Input: dimensioned drawing with shaded views. Units: mm. Origin: part minimum x, y, z. A direction names the side the tool comes from. Give positions to 0.01 mm unless a question says otherwise; leave off trailing zeros. Write each loop counter-clockwise with the first axis right and the second up, starting at its lowest first coordinate (ties: lowest second). Pieces come first, ordered by that corner, then holes. Notation, with made-up numbers: (4, 78.5) - (48, 78.5) arc R14 cw to (48, 102.5) - close; hole circle Ø4 at (39, 41.5). An arc over 180 degrees is marked (long way). Answer as CSV lines item,"result".
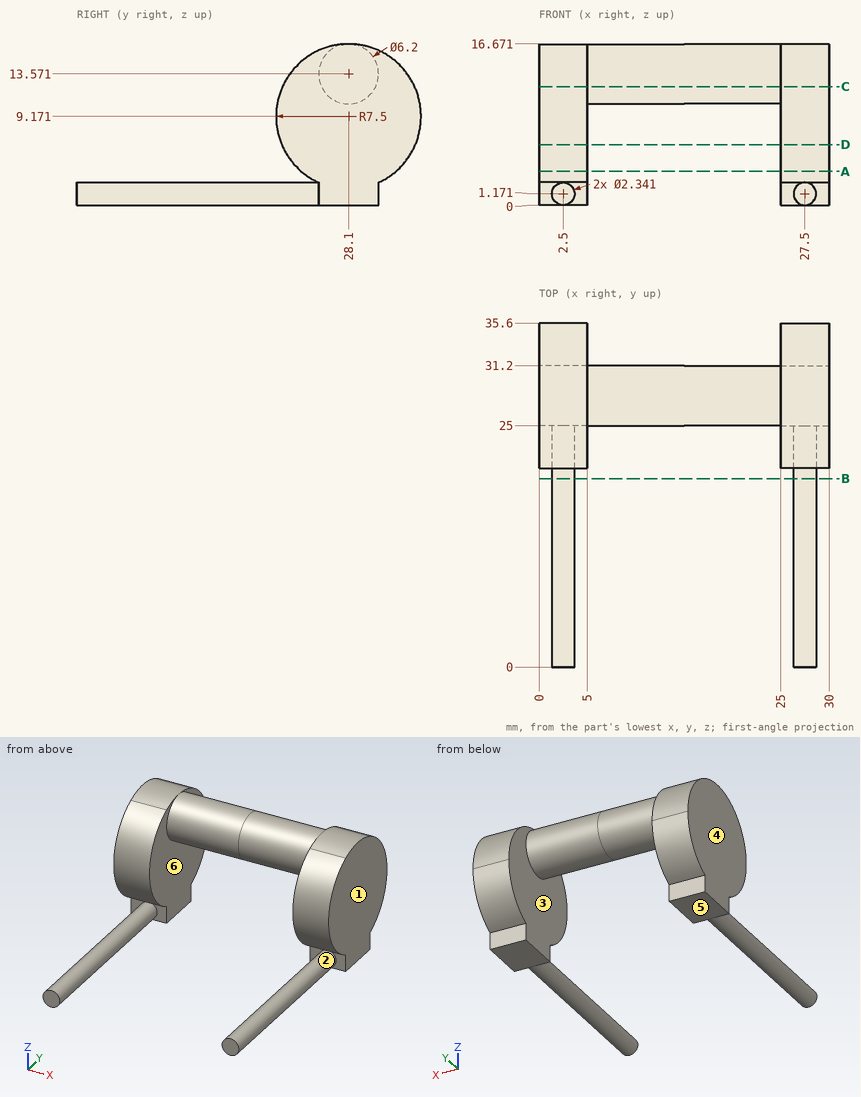
Item 1: Cut plane B-B on y = 19.5. Return the cut outline in (x, z).
The answers:
outline,"circle Ø2.34 at (2.5, 1.17); circle Ø2.34 at (27.5, 1.17)"
Item 2: Mould query, pull axis X, two halves, no side actions, for the marked faces 3, 4, 5 and 6. Classes: +X half, -X half, draft (parallel to the pull), parting line (faces both ways), or undercut.
The answers:
face 3,"undercut"
face 4,"-X half"
face 5,"draft"
face 6,"undercut"
Item 3: Cut plane D-D on z = 6.25. Return the cut outline in (x, y).
The answers:
outline,"(0, 21.19) - (5, 21.19) - (5, 35.01) - (0, 35.01) - close; (25, 21.19) - (30, 21.19) - (30, 35.01) - (25, 35.01) - close"
Item 4: Reachability of the marked faces 1 and 2 from +Z, -Z, +X, -X, +Y, -Y: full face, straight path, thin tool, end or side. Return the list, or none.
The answers:
face 1,"+Z, -Z, +X, +Y, -Y"
face 2,"-Y"
Item 5: Contact query for flat-ended pins moving along their axis: pin 1 (2.5 mm diameter, centred on x = 3, z = 1.5, fed in from +Y) (1 decimal); pin 2 (8 mm diameter, centred on y = 9.5, z = 5.5, fed in from -X); pin 3 (0.7 mm diameter, centred on x = 27.5, z = 1, fed in from +Y). Output: stop coordinate, or through.
The answers:
pin 1,"y = 32"
pin 2,"x = 1.38"
pin 3,"y = 31.2"
Item 6: Cut plane C-C on z = 12.25. Return the cut outline in (x, y) (1 decimal).
The answers:
outline,"(0, 21.3) - (5, 21.3) - (5, 25.3) - (25, 25.3) - (25, 21.3) - (30, 21.3) - (30, 34.9) - (25, 34.9) - (25, 30.9) - (5, 30.9) - (5, 34.9) - (0, 34.9) - close"
Item 7: Cut plane A-A on z = 3.5. Return the cut outline in (x, y).
The answers:
outline,"(0, 23.19) - (5, 23.19) - (5, 33.01) - (0, 33.01) - close; (25, 23.19) - (30, 23.19) - (30, 33.01) - (25, 33.01) - close"
Item 8: Ray query, line 1 (X direction, y = 32.5, z = 4); line 2 (Z direction, x = 27.5, y = 3); line 3 (Y direction, x = 3, z = 6.5). Return the intervals inside material, ascending. Write a range as from..to.
The answers:
line 1,"0..5, 25..30"
line 2,"0..2.34"
line 3,"21.09..35.11"
